```python
from build123d import *

# Parameters (mm, degrees)
F0_W      = 127
F0_H      = 101.6
F1_DEPTH  = 190.5
F2_T      = -2.54
F10_E18_W = 60.96
F10_E18_H = 190.5
F19_DEPTH = 2.54
F12_E19_W = 77.7505575543
F12_E19_H = 190.5
F20_DEPTH = 2.54
F14_E20_W = 48.26
F14_E20_H = 190.5
F21_DEPTH = 2.54
F16_E21_W = 77.7505575543
F16_E21_H = 190.5
F22_DEPTH = 2.54
F18_E22_W = 60.96
F18_E22_H = 190.5
F23_DEPTH = 2.54
F4_E9_W   = 77.7505575543
F4_E9_H   = 187.96
F24_DEPTH = 2.54
F6_E16_W  = 48.26
F6_E16_H  = 190.5
F25_DEPTH = 2.54
F8_E17_W  = 77.7505575543
F8_E17_H  = 190.5
F26_DEPTH = 2.54


with BuildPart() as f1:
    # F0 (on Top) → F1 (new body)
    with BuildSketch(Plane.XY):
        Rectangle(F0_W, F0_H)
    extrude(amount=F1_DEPTH)

    # F2
    f2_openings = [f1.faces().sort_by_distance(p)[0] for p in [
        (0, 0, 190.5),
    ]]
    offset(amount=F2_T, openings=f2_openings)

    # F10_E18 (on explicit) → F19 (join)
    with BuildSketch(Plane(origin=(0, 0, 2.54), x_dir=(-1, 0, 0), z_dir=(0, 1, 0))):
        with Locations((30.48, 95.25)):
            Rectangle(F10_E18_W, F10_E18_H)
    extrude(amount=F19_DEPTH)

    # F12_E19 (on explicit) → F20 (join)
    with BuildSketch(Plane(origin=(0, 0, 2.54), x_dir=(-0.7840458245, -0.6207029444, 0), z_dir=(-0.6207029444, 0.7840458245, 0))):
        with Locations((38.8752787771, 95.25)):
            Rectangle(F12_E19_W, F12_E19_H)
    extrude(amount=F20_DEPTH)

    # F14_E20 (on explicit) → F21 (join)
    with BuildSketch(Plane(origin=(0, 0, 2.54), x_dir=(0, -1, 0), z_dir=(-1, 0, 0))):
        with Locations((24.13, 95.25)):
            Rectangle(F14_E20_W, F14_E20_H)
    extrude(amount=F21_DEPTH)

    # F16_E21 (on explicit) → F22 (join)
    with BuildSketch(Plane(origin=(0, 0, 2.54), x_dir=(0.7840458245, -0.6207029444, 0), z_dir=(-0.6207029444, -0.7840458245, 0))):
        with Locations((38.8752787771, 95.25)):
            Rectangle(F16_E21_W, F16_E21_H)
    extrude(amount=F22_DEPTH)

    # F18_E22 (on explicit) → F23 (join)
    with BuildSketch(Plane(origin=(0, 0, 2.54), x_dir=(1, 0, 0), z_dir=(0, -1, 0))):
        with Locations((30.48, 95.25)):
            Rectangle(F18_E22_W, F18_E22_H)
    extrude(amount=F23_DEPTH)

    # F4_E9 (on explicit) → F24 (join)
    with BuildSketch(Plane(origin=(60.96, 48.26, 2.54), x_dir=(-0.7840458245, -0.6207029444, 0), z_dir=(-0.6207029444, 0.7840458245, 0))):
        with Locations((38.8752787771, 93.98)):
            Rectangle(F4_E9_W, F4_E9_H)
    extrude(amount=F24_DEPTH)

    # F6_E16 (on explicit) → F25 (join)
    with BuildSketch(Plane(origin=(0, 0, 2.54), x_dir=(0, 1, 0), z_dir=(1, 0, 0))):
        with Locations((24.13, 95.25)):
            Rectangle(F6_E16_W, F6_E16_H)
    extrude(amount=F25_DEPTH)

    # F8_E17 (on explicit) → F26 (join)
    with BuildSketch(Plane(origin=(-60.96, 48.26, 2.54), x_dir=(0.7840458245, -0.6207029444, 0), z_dir=(-0.6207029444, -0.7840458245, 0))):
        with Locations((38.8752787771, 95.25)):
            Rectangle(F8_E17_W, F8_E17_H)
    extrude(amount=F26_DEPTH)


solid = f1.part
```
For this review, take the finished solid that the model builds, in its own axes (mm). A direction names the side the tool comes from. Round coordinates to 2 decimals unless told otherwise and drop trailing zeros. Write each loop counter-clockwise with the first axis right and the second up, starting at its lowest first coordinate (ties: lowest second). Pieces come first, ordered by that corner, then holes. Notation, with made-up numbers: (26.25, 45) -> (49.25, 45) arc R19 ccw to (49.25, 79) -> close; hole circle Ø2 at (69.25, -31.5). An arc over 180 degrees is marked (long way). Use one line per item in the form item = value.
Q1. To check wall thickness, follow probe 1 along Y at (x, z) = (-4, 56); probe 2 along Y at (x, z) = (-51, 126.5) (3 decimals); probe 3 along Y at (x, z) = (42.5, 184). State the ranges of each line that lie inside material, in increasing order. Write a range as from..to.
Resolved:
probe_1 = -50.8..-48.26, -3.17..3.17, 48.26..50.8
probe_2 = -50.8..-48.26, -40.375..-37.135, 0..2.54, 37.135..40.375, 48.26..50.8
probe_3 = -50.8..-48.26, -36.89..-33.65, -2.54..0, 33.65..36.89, 48.26..50.8
Q2. Consider section B-B (x = 41). State the section outline as (y, z) points.
Resolved:
outline = (-50.8, 0) -> (50.8, 0) -> (50.8, 190.5) -> (48.26, 190.5) -> (48.26, 2.54) -> (35.7, 2.54) -> (35.7, 190.5) -> (32.46, 190.5) -> (32.46, 2.54) -> (0, 2.54) -> (0, 193.04) -> (-2.54, 193.04) -> (-2.54, 2.54) -> (-32.46, 2.54) -> (-32.46, 193.04) -> (-35.7, 193.04) -> (-35.7, 2.54) -> (-48.26, 2.54) -> (-48.26, 190.5) -> (-50.8, 190.5) -> close
Q3. Consider section A-A (z = 110.5). State how many separate pieces and enclosed holes the cut face has, then the cut area to 3 significant figures.
Resolved:
separate_pieces = 1
enclosed_holes = 8
area = 2,430 mm²
Q4. The part is to be moulded in two halves that separate along X. For faces 3 (the flat face through (63.5, -1, 94)), 4 (the flat face through (-60.96, -23, 95)), 5 (the flat face through (-1, 0, 193.04)), say which applies: released by +X, released by -X, zero draft, split by the parting line, or undercut.
Resolved:
face_3 = released by +X
face_4 = undercut
face_5 = zero draft
Q5. Clearance check with flat-ended pins moving along their axes: pin 1 Ø0.8 at (x, z) = (0.5, 192) entering from +Y; pin 2 Ø12 at (x, y) = (48, 25.5) entering from +Z; pin 3 Ø0.6 at (x, y) = (-0.5, 3) entering from +Z. State where each tip first meets the part, or that it passes through.
Resolved:
pin_1 = 48.26
pin_2 = 2.54
pin_3 = 190.5
Q6. Machinability: for faces 1 (the flat face through (-2.54, -25, 99)), 2 (the flat face through (-1, 50.8, 94)), which of the approach directions +Z, -Z, +X, -X, +Y, -Y give a long, thin tool a straight path to every point of the face, cutting with its end or side? Answer none if there is none.
Resolved:
face_1 = +Z
face_2 = +Z, -Z, +X, -X, +Y
Q7. Consider section C-C (y = -41.5). State the section outline as (x, z) points, then the cut area to 3 significant figures.
Resolved:
outline = (-63.5, 0) -> (63.5, 0) -> (63.5, 190.5) -> (60.96, 190.5) -> (60.96, 2.54) -> (52.42, 2.54) -> (52.42, 193.04) -> (48.33, 193.04) -> (48.33, 2.54) -> (0, 2.54) -> (0, 193.04) -> (-2.54, 193.04) -> (-2.54, 2.54) -> (-52.42, 2.54) -> (-52.42, 193.04) -> (-56.51, 193.04) -> (-56.51, 2.54) -> (-60.96, 2.54) -> (-60.96, 190.5) -> (-63.5, 190.5) -> close
area = 3,320 mm²
